Can you work these out from the drawing? Everything is in mm from the part's minimum corner. Round coordinates to 2 decimals unless told otherwise and drop trailing zeros. Order: outer loops, then holes, each group sorted by start corner. A loop starts at its lowest first (then second) coordinate and runs counter-clockwise, first axis right, second up. Notation, with made-up numbers: M 86,46 L 145,46 A18 ccw 145,80 Z; hole C 86,8 d11. An arc over 180 degrees is marked long. Write item = value, one per line. Start each with the question number.
Item 1: I want a section at A-A, the plane x = 15. List the corners of the cut face in (y, z) for me.
Item 2: I want a section at B-B, the plane z = 15.5. List the corners of the cut face in (x, y) for me, plus the area to 3 significant figures.
Item 3: I want a section at C-C, the plane x = 23.5. List the corners of the cut face in (y, z) for me.
Item 4: Please list where these lines run through material, in increasing order: L1, parallel to Y at x = 19, z = 14; L2, parallel to X at y = 107.5, z = 16.5; L3, parallel to Y at x = 13, z = 16.
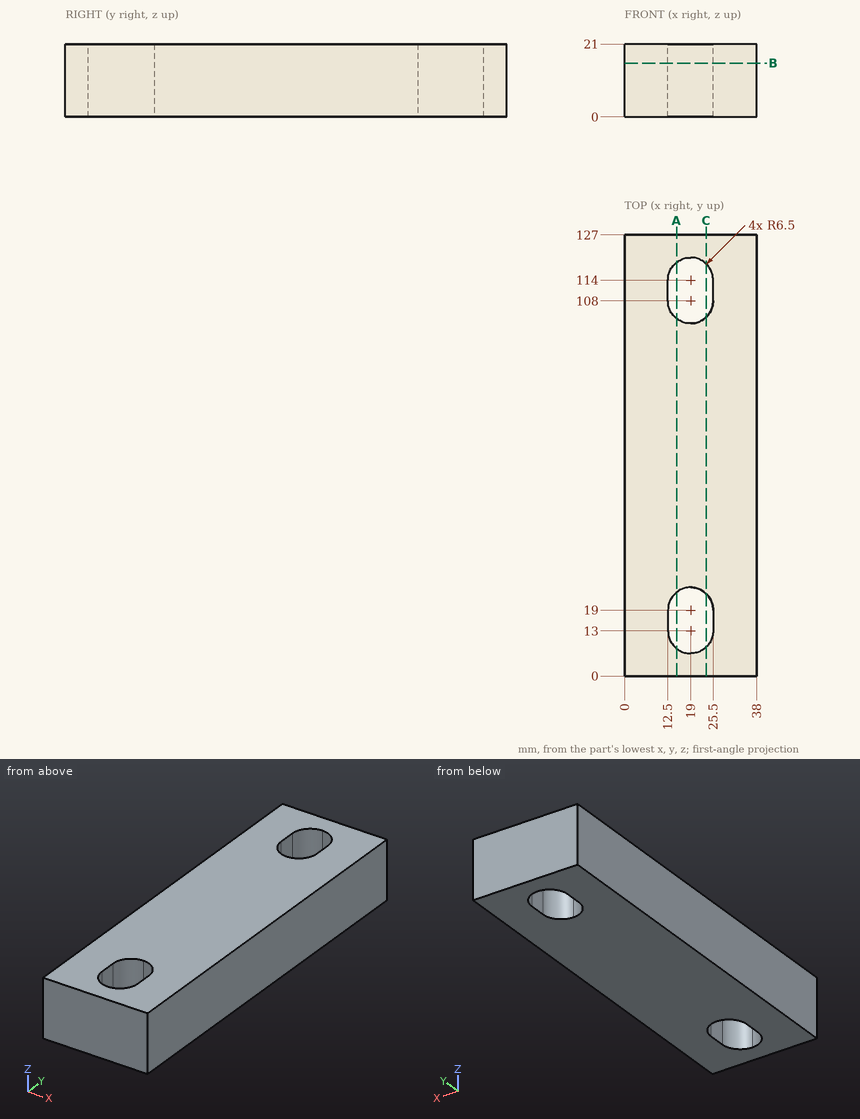
Filled in:
q1.outline = M 0,0 L 7.88,0 L 7.88,21 L 0,21 Z; M 24.12,0 L 102.88,0 L 102.88,21 L 24.12,21 Z; M 119.12,0 L 127,0 L 127,21 L 119.12,21 Z
q2.outline = M 0,0 L 38,0 L 38,127 L 0,127 Z; hole M 12.5,13 A6.5 ccw 25.5,13 L 25.5,19 A6.5 ccw 12.5,19 Z; hole M 12.5,108 A6.5 ccw 25.5,108 L 25.5,114 A6.5 ccw 12.5,114 Z
q2.area = 4,400 mm^2
q3.outline = M 0,0 L 8.31,0 L 8.31,21 L 0,21 Z; M 23.69,0 L 103.31,0 L 103.31,21 L 23.69,21 Z; M 118.69,0 L 127,0 L 127,21 L 118.69,21 Z
q4.L1 = 0 to 6.5, 25.5 to 101.5, 120.5 to 127
q4.L2 = 0 to 12.52, 25.48 to 38
q4.L3 = 0 to 10.5, 21.5 to 105.5, 116.5 to 127
